CAD build for the part. Positions are in the model's coordinates, mm. Give positions to 0.01 mm unless a question says otherwise; leave off trailing zeros. Write each loop counter-clockwise with the first axis right and the second up, starting at its lowest first coordinate (ties: lowest second). Pieces come first, ordered by that corner, then holes. Notation, with made-up numbers: (76, 5.25) - (119, 5.25) arc R23 ccw to (119, 25.25) - close; hole circle Ø8 at (-4, -10.5). An arc over 180 degrees is marked (long way). Answer as a JSON object with one key per item and string values.
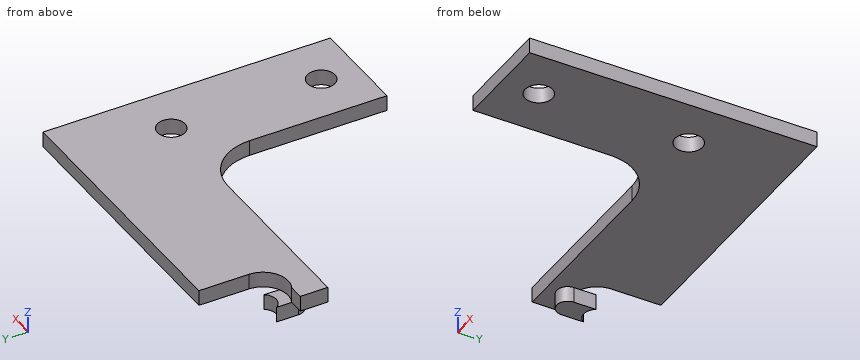
Autodesk Inventor part; units mm, degrees
ref_plane "Work Plane5" through (0, 0, 0) normal (0, 0, 1) x (1, 0, 0)
ref_plane "Work Plane6" through (0, 0, 0) normal (0, 0, 1) x (1, 0, 0)
ref_plane "YZ Plane" through (0, 0, 0) normal (1, 0, 0) x (0, 1, 0)
ref_plane "Work Plane5" through (0, 0, 0) normal (0, 0, 1) x (1, 0, 0)
sketch "Sketch1" plane through (0, 0, 0) normal (0, 0, 1) x (1, 0, 0)
  arc A0 (-50, 35.3137) -> (-46, 35.3137) centre (-48, 35.3137) ccw construction
  arc A1 (-46, 40) -> (-50, 40) centre (-48, 40) ccw construction
  line L0 (-50, 35.3137) -> (-50, 40) construction
  line L1 (-46, 40) -> (-46, 35.3137) construction
  line L2 (-46.254, 38.8332) -> (-46.254, 35.3137)
  arc A2 (-49.746, 35.3137) -> (-46.254, 35.3137) centre (-48, 35.3137) ccw
  line L3 (-49.746, 35.3137) -> (-49.746, 38.8332)
  arc A3 (-49.746, 38.8332) -> (-46.254, 38.8332) centre (-48, 40) ccw
  point P0 (0, 0)
  dimension "d1" = 4.2
extrude "Extrusion1" add sketch "Sketch1" against normal blind 2.5
ref_plane "Work Plane6" through (0, 0, 0) normal (0, 0, 1) x (1, 0, 0)
sketch "Sketch2" plane through (0, 0, 0) normal (0, 0, 1) x (1, 0, 0)
  line L0 (-52.1646, 48) -> (0, 48)
  line L1 (0, 48) -> (0, 2)
  arc A0 (-16, 24) -> (-24, 32) centre (-24, 24) ccw
  circle A1 centre (-8, 8) radius 2.2
  circle A2 centre (-8, 32) radius 2.2
  line L2 (-52.1646, 32) -> (-24, 32)
  line L3 (-16, 24) -> (-16, 2)
  line L4 (0, 2) -> (-16, 2)
  arc A3 (-49.746, 38.8332) -> (-46.254, 38.8332) centre (-48, 40) ccw
  line L5 (-52.1646, 48) -> (-52.1646, 32)
  line L6 (-52.1646, 48) -> (-36.1646, 48) construction
  point P0 (-54, 48)
  dimension "d7" = 4.4
  dimension "d8" = 4.4
  dimension "d9" = 24
  dimension "d22" = 48
  dimension "d23" = 90
  dimension "d24" = 46
  dimension "d25" = 16
  dimension "d26" = 8
  dimension "d27" = 8
extrude "Extrusion2" add sketch "Sketch2" along normal blind 2.5
sketch "Sketch6" plane through (0, 0, 0) normal (0, 0, -1) x (-1, 0, 0)
  arc A0 (46.254, 38.8332) -> (49.746, 38.8332) centre (48, 40) ccw
  arc A1 (44, 40) -> (49.746, 36.4012) centre (48, 40) ccw
  line L0 (52.1646, 48) -> (52.1646, 32)
  line L1 (49.746, 35.3137) -> (49.746, 38.8332)
  line L2 (49.746, 36.4012) -> (52.1646, 36.4012)
  line L3 (52.1646, 36.4012) -> (52.1646, 44)
  line L4 (44, 40) -> (44, 48)
  line L5 (0, 48) -> (52.1646, 48)
  line L6 (44, 48) -> (52.1646, 48)
  line L7 (52.1646, 44) -> (52.1646, 48)
  point P0 (0, 0)
  dimension "d31" = 8
extrude "Extrusion6" cut sketch "Sketch6" against normal up to surface (2.5 mm away)
properties part number "Odometry stop left"
(1) Saw through at C-C, the plane x = -8. Give the cut face in (y, z).
Answer key:
{"outline": "(2, 0) - (5.8, 0) - (5.8, 2.5) - (2, 2.5) - close; (10.2, 0) - (29.8, 0) - (29.8, 2.5) - (10.2, 2.5) - close; (34.2, 0) - (48, 0) - (48, 2.5) - (34.2, 2.5) - close"}
(2) Saw through at D-D, the plane x = -48. Give the cut face in (y, z), and give its area (3 significant figures).
Answer key:
{"outline": "(32, 0) - (33.57, 0) - (33.57, -2.5) - (37.9, -2.5) - (37.9, 0) - (36, 0) - (36, 2.5) - (32, 2.5) - close", "area": "20.8 mm²"}
(3) Flat gauge pins, fed straight in: P1, Ø7, axis at x = -8, y = 32, coming from the -Z side; P2, Ø1.2, axis at y = 11.5, z = 1.5, coming from the -X side; P3, Ø1.2, axis at y = 36.5, z = -1.5, coming from the -X side. Where does each tip first touch, or does it go through?
Answer key:
{"P1": "stops at z = 0", "P2": "stops at x = -16", "P3": "stops at x = -49.75"}
(4) Saw through at B-B, the plane z = 0.85. Give the cut face in (x, y), and give its area (3 significant figures).
Answer key:
{"outline": "(-52.16, 32) - (-24, 32) arc R8 cw to (-16, 24) - (-16, 2) - (0, 2) - (0, 48) - (-44, 48) - (-44, 40) arc R4 cw to (-49.75, 36.4) - (-52.16, 36.4) - close; hole circle Ø4.4 at (-8, 8); hole circle Ø4.4 at (-8, 32)", "area": "1,200 mm²"}
(5) Saw through at A-A, the plane y = 8. Give the cut face in (x, z), and give its area (3 significant figures).
Answer key:
{"outline": "(-16, 0) - (-10.2, 0) - (-10.2, 2.5) - (-16, 2.5) - close; (-5.8, 0) - (0, 0) - (0, 2.5) - (-5.8, 2.5) - close", "area": "29.0 mm²"}
(6) Probe L1, parallel to Y at x = -8, z = 0.95; L2, parallel to Z at x = -12, y = 39; L3, parallel to X at y = 30, z = 2.1. List the from-to ranges inside material, lowest first. Write a range as [from, to].
Answer key:
{"L1": "y = [2, 5.8], [10.2, 29.8], [34.2, 48]", "L2": "z = [0, 2.5]", "L3": "x = [-18.71, -8.92], [-7.08, 0]"}
